Verification items for the finished model (mm, model axes). Round coordinates to 2 decimals unless told otherwise and drop trailing zeros. Write each loop counter-clockwise with the first axis right and the second up, starting at its lowest first coordinate (ties: lowest second). Pieces come first, ordered by that corner, then holes. Notation, with made-up numbers: (56, 64.25) - (108, 64.25) arc R20 cw to (108, 100.25) - close; hole circle Ø8 at (60, -21.75). An arc over 180 degrees is marked (long way). Write each question's results on one line, items separated by ' | '.
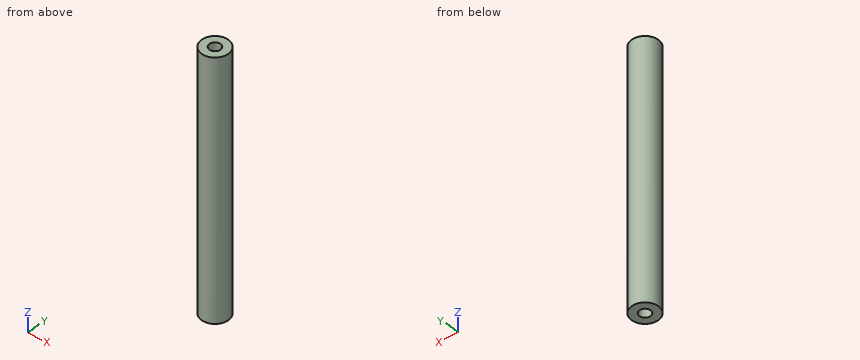
Autodesk Inventor part; units mm, degrees
ref_plane "YZ Plane" through (0, 0, 0) normal (1, 0, 0) x (0, 1, 0)
ref_plane "XZ Plane" through (0, 0, 0) normal (0, 1, 0) x (-1, 0, 0)
sketch "Sketch1" plane through (0, 0, 0) normal (0, 0, 1) x (1, 0, 0)
  circle A0 centre (0, 0) radius 4.445
  dimension "d1" = 8.89
extrude "Extrusion1" add sketch "Sketch1" along normal mid plane 84.9884
ref_plane "Work Plane1" through (0, 0, 0) normal (0, 0, 1) x (1, 0, 0)
sketch "Sketch2" plane through (0, 0, 42.4942) normal (0, 0, 1) x (1, 0, 0)
  point P0 (0, 0)
hole "Hole1" at (0, 0, 42.4942) direction (0, 0, -1) diameter 3.683 depth 14.9352 tip angle 118
mirror "Mirror1" about plane through (0, 0, 0) normal (0, 0, 1) of "Hole1"
properties part number "drive train standoff"
(1) Go/stop test with flat-tipped pins: pin 1 Ø2 at (x, z) = (-1.5, 26.5) entering from -Y; pin 2 Ø2 at (x, y) = (0, 0) entering from +Z; pin 3 Ø3 at (x, y) = (0, 0) entering from -Z. Record where each tip stops, or that it passes through.
Answer:
pin 1: y = -4.42 | pin 2: z = 27.05 | pin 3: z = -27.35
(2) Section check A-A (z = 34.5). Record the cut outline in (x, y) (1 decimal).
Answer:
outline: circle Ø8.9 at (0, 0); hole circle Ø3.7 at (0, 0)
(3) Section check C-C (x = -3.5). Record the cut outline in (y, z).
Answer:
outline: (-2.74, -42.49) - (2.74, -42.49) - (2.74, 42.49) - (-2.74, 42.49) - close
(4) Section check B-B (z = -23). Record the cut outline in (x, y) (3 decimals), plus the area to 3 significant figures.
Answer:
outline: circle Ø8.89 at (0, 0) | area: 62.1 mm2
(5) Thickness scan on L1, parallel to Y at x = 0, z = 32 (1 decimal); L2, parallel to X at y = -0.25, z = 25; L3, parallel to Y at x = -2.5, z = 31. Record the ranges inside material, lowest first.
Answer:
L1: -4.4 to -1.8, 1.8 to 4.4 | L2: -4.44 to 4.44 | L3: -3.68 to 3.68
